Model file for the job. Use its own axes, mm. Coordinates: 2 decimals unless noted, no trailing zeros. Order: outer loops, then holes, each group sorted by start corner. A loop starts at its lowest first (then second) coordinate and runs counter-clockwise, first axis right, second up. Notation, with made-up numbers: M -14,86.25 L 21,86.25 A28 cw 21,114.25 Z; hole C 41,25.5 d4. An arc over 180 degrees is marked long. Return JSON: item names as keys, results as strings.
```python
from build123d import *

# Parameters (mm, degrees)
F0_R     = 15.24
F1_DEPTH = 12.7
F2_R     = 13.97
F3_DEPTH = 12.7
F4_R     = 13.97
F5_DEPTH = 12.7


with BuildPart() as f1:
    # F0 (on Top) → F1 (new body)
    with BuildSketch(Plane.XY):
        Circle(F0_R)
    extrude(amount=F1_DEPTH)

    # F2 (on Top) → F3 (cut)
    with BuildSketch(Plane.XY):
        with Locations((-10.602972, 18.632865)):
            Circle(F2_R)
    extrude(amount=-F3_DEPTH, mode=Mode.SUBTRACT)

    # F4 (on Top) → F5 (cut)
    with BuildSketch(Plane.XY):
        Circle(F4_R)
    extrude(amount=F5_DEPTH, mode=Mode.SUBTRACT)


solid = f1.part
```
Item 1: Saw through at A-A (x = 0). Write the cut outline in (y, z).
Check result:
{"outline": "M -15.24,0 L -13.97,0 L -13.97,12.7 L -15.24,12.7 Z; M 13.97,0 L 15.24,0 L 15.24,12.7 L 13.97,12.7 Z"}
Item 2: Wall check: line 1 (Y direction, x = 0, z = 5.75); line 2 (Y direction, x = -10, z = 11.5); line 3 (X direction, y = -12.5, z = 2.75). Give the ranges that are in metal, low to high.
Check result:
{"line 1": "y = -15.24 to -13.97, 13.97 to 15.24", "line 2": "y = -11.5 to -9.76, 9.76 to 11.5", "line 3": "x = -8.72 to -6.24, 6.24 to 8.72"}
Item 3: Drop flat-ended pins along their axis: pin 1 Ø4 at (y, z) = (2.5, 4.5) entering from +X; pin 2 Ø1 at (y, z) = (-0.5, 7) entering from -X; pin 3 Ø1 at (y, z) = (4.5, 9) entering from +X. Give the stop position or say it passes through.
Check result:
{"pin 1": "stops at x = 15.23", "pin 2": "stops at x = -15.24", "pin 3": "stops at x = 14.71"}
Item 4: Saw through at B-B (y = -5.5). Write the cut outline in (x, z), and give its area (3 significant figures).
Check result:
{"outline": "M -14.21,0 L -12.84,0 L -12.84,12.7 L -14.21,12.7 Z; M 12.84,0 L 14.21,0 L 14.21,12.7 L 12.84,12.7 Z", "area": "34.8 mm2"}
Item 5: Saw through at C-C (z = 8.5). Write the cut outline in (x, y).
Check result:
{"outline": "C 0,0 d30.48; hole C 0,0 d27.94"}
